Could you check a few things on this model? Use its own coordinates, in mm. Face numbers are marked on the shaded views. A direction names the side the tool comes from. Give positions to 0.01 mm unless a question says otherwise; leave off trailing zeros. Order: outer loops, then holes, each group sorted by start corner. A loop starts at its lowest first (then second) coordinate and runs counter-clockwise, first axis right, second up. Notation, with made-up numbers: M 62,10 L 99,10 A23 ccw 99,44 Z; hole C -29.75,48.5 d11. An arc over 180 degrees is marked long. Use a Markdown table: item, result. Add a question column.
Item 1: If I drill on L1, parallel to X at y = 116, z = 4.25; L2, parallel to X at y = 117, z = 8.05; L3, parallel to Y at x = 6, z = 5.25, over which ranges is the centre line in solid material (lowest first)? Write a range as from..to.
Item 2: Suppose I cut it at D-D on x = -4.25. Write out the boundary of the cut face in (y, z), plus the area to 3 significant figures.
Item 3: Suppose I cut it at A-A on x = 7. Write out the boundary of the cut face in (y, z).
Item 4: I'm going to push flat-ended pins straight in: pin 1 Ø1.5 at (x, y) = (6.5, 118) entering from +Z; pin 2 Ø2 at (x, z) = (-5.5, 7.5) entering from -Y; pin 3 Ø1 at (y, z) = (123, 4.5) entering from -X. Where does each tip first touch, or does it pass through?
Item 5: If we mould it in two halves opening along X, with no side actions, what happens to the marked faces 1, 2 and 3? For each: released by +X, released by -X, zero draft, split by the parting line, or undercut.
Item 6: Suppose I cut it at B-B on y = 118.25. Write out the boundary of the cut face in (x, z), plus the area to 3 significant figures.
Item 7: Suppose I cut it at C-C on z = 1.75. Write out the boundary of the cut face in (x, y), plus the area to 3 significant figures.
Item 8: For the marked faces 4 and 5, which set-ups out of +Z, -Z, +X, -X, +Y, -Y let a thin tool reach every point of the face, with its end or its side?
from build123d import *

# Parameters (mm, degrees)
CYLINDER568_R               = 3
CYLINDER568_DEPTH           = 4
CYLINDER569_R               = 3
CYLINDER569_DEPTH           = 4
CYLINDER563_R               = 3
CYLINDER563_DEPTH           = 4
CYLINDER570_R               = 3
CYLINDER570_DEPTH           = 4
COMPOUND332_PLACEMENT_ANGLE = 90
CYLINDER566_R               = 1.5
CYLINDER566_DEPTH           = 20
CYLINDER565_R               = 1.5
CYLINDER565_DEPTH           = 20
CYLINDER567_R               = 1.5
CYLINDER567_DEPTH           = 20
CYLINDER564_R               = 1.5
CYLINDER564_DEPTH           = 20
COMPOUND333_PLACEMENT_ANGLE = 90
CYLINDER534_R               = 10
CYLINDER534_DEPTH           = 10


with BuildPart() as obj1:
    # Cylinder568 → Cylinder568 (new body)
    with BuildSketch(Plane(origin=(-7, -34, 37), x_dir=(1, 0, 0), z_dir=(0, -1, 0))):
        Circle(CYLINDER568_R)
    extrude(amount=CYLINDER568_DEPTH)


with BuildPart() as obj2:
    # Cylinder569 → Cylinder569 (new body)
    with BuildSketch(Plane(origin=(7, -34, 73), x_dir=(1, 0, 0), z_dir=(0, -1, 0))):
        Circle(CYLINDER569_R)
    extrude(amount=CYLINDER569_DEPTH)


with BuildPart() as obj3:
    # Cylinder563 → Cylinder563 (new body)
    with BuildSketch(Plane(origin=(-7, -34, 73), x_dir=(1, 0, 0), z_dir=(0, -1, 0))):
        Circle(CYLINDER563_R)
    extrude(amount=CYLINDER563_DEPTH)


with BuildPart() as compound332:
    # Cylinder570 → Cylinder570 (new body)
    with BuildSketch(Plane(origin=(7, -34, 37), x_dir=(1, 0, 0), z_dir=(0, -1, 0))):
        Circle(CYLINDER570_R)
    extrude(amount=CYLINDER570_DEPTH)

    # Compound332: union obj1, obj2, obj3
    add(obj1.part)
    add(obj2.part)
    add(obj3.part)


with BuildPart() as compound332_1:
    # Compound332 placement: moved
    add(compound332.part.moved(Location((0, 141, 45))).rotate(Axis((0, 141, 45), (1, 0, 0)), COMPOUND332_PLACEMENT_ANGLE))


with BuildPart() as obj4:
    # Cylinder566 → Cylinder566 (new body)
    with BuildSketch(Plane(origin=(-7, -34, 37), x_dir=(1, 0, 0), z_dir=(0, -1, 0))):
        Circle(CYLINDER566_R)
    extrude(amount=CYLINDER566_DEPTH)


with BuildPart() as obj5:
    # Cylinder565 → Cylinder565 (new body)
    with BuildSketch(Plane(origin=(7, -34, 73), x_dir=(1, 0, 0), z_dir=(0, -1, 0))):
        Circle(CYLINDER565_R)
    extrude(amount=CYLINDER565_DEPTH)


with BuildPart() as obj6:
    # Cylinder567 → Cylinder567 (new body)
    with BuildSketch(Plane(origin=(-7, -34, 73), x_dir=(1, 0, 0), z_dir=(0, -1, 0))):
        Circle(CYLINDER567_R)
    extrude(amount=CYLINDER567_DEPTH)


with BuildPart() as compound333:
    # Cylinder564 → Cylinder564 (new body)
    with BuildSketch(Plane(origin=(7, -34, 37), x_dir=(1, 0, 0), z_dir=(0, -1, 0))):
        Circle(CYLINDER564_R)
    extrude(amount=CYLINDER564_DEPTH)

    # Compound333: union obj4, obj5, obj6
    add(obj4.part)
    add(obj5.part)
    add(obj6.part)


with BuildPart() as compound333_1:
    # Compound333 placement: moved
    add(compound333.part.moved(Location((0, 141, 45))).rotate(Axis((0, 141, 45), (1, 0, 0)), COMPOUND333_PLACEMENT_ANGLE))


with BuildPart() as cut190:
    # Cylinder534 → Cylinder534 (new body)
    with BuildSketch(Plane(origin=(0, 106, 0), x_dir=(1, 0, 0), z_dir=(0, 0, 1))):
        Circle(CYLINDER534_R)
    extrude(amount=CYLINDER534_DEPTH)

    # Cut189: cut Compound333
    add(compound333_1.part, mode=Mode.SUBTRACT)

    # Cut190: cut Compound332
    add(compound332_1.part, mode=Mode.SUBTRACT)


with BuildPart() as cut190_1:
    # Cut190 placement: moved
    add(cut190.part.moved(Location((0, 13, 0))))


solid = cut190_1.part
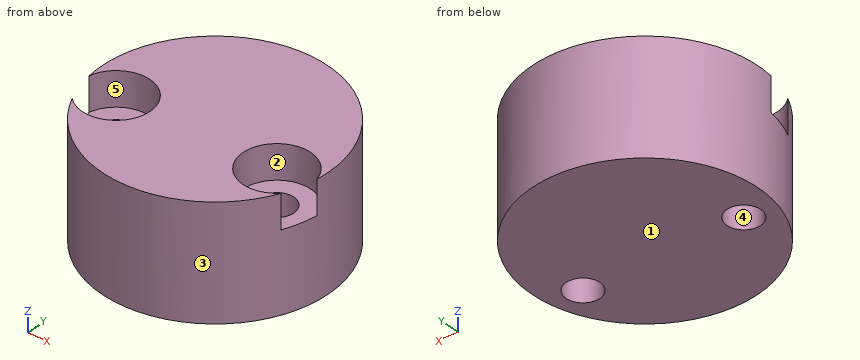
Findings below:
| question | item | result |
|---|---|---|
| 1 | L1 | x = -9.54..-8.12, -5.88..5.88, 8.12..9.54 |
| 1 | L2 | x = -4..4 |
| 1 | L3 | y = 111..115.88, 118.12..127 |
| 2 | outline | M 109.95,0 L 128.05,0 L 128.05,10 L 118.2,10 L 118.2,7 L 115.8,7 L 115.8,10 L 109.95,10 Z |
| 2 | area | 174 mm^2 |
| 3 | outline | M 111.86,0 L 115.5,0 L 115.5,7 L 114,7 L 114,10 L 111.86,10 Z; M 118.5,0 L 126.14,0 L 126.14,10 L 120,10 L 120,7 L 118.5,7 Z |
| 4 | pin 1 | stops at z = 7 |
| 4 | pin 2 | stops at y = 110.07 |
| 4 | pin 3 | stops at x = -9.37 |
| 5 | face 1 | zero draft |
| 5 | face 2 | undercut |
| 5 | face 3 | split by the parting line |
| 6 | outline | M -9.97,0 L -7.83,0 L -7.83,7 L -9.73,7 L -9.73,10 L -9.97,10 Z; M -6.17,0 L 6.17,0 L 6.17,7 L 4.27,7 L 4.27,10 L -4.27,10 L -4.27,7 L -6.17,7 Z; M 7.83,0 L 9.97,0 L 9.97,10 L 9.73,10 L 9.73,7 L 7.83,7 Z |
| 6 | area | 143 mm^2 |
| 7 | outline | C 0,119 d20; hole C -7,117 d3; hole C 7,117 d3 |
| 7 | area | 300 mm^2 |
| 8 | face 4 | +Z, -Z |
| 8 | face 5 | +Z |
